Part model, mm, in its own coordinate system. Round coordinates to 2 decimals unless told otherwise and drop trailing zeros. Write each loop counter-clockwise with the first axis right and the second up, starting at its lowest first coordinate (ties: lowest second). Pieces come first, ordered by that corner, then holes. Notation, with made-up numbers: M 19,-36.75 L 48,-36.75 A22 ccw 48,-26.75 Z; hole C -17,84 d10. An arc over 180 degrees is marked long. Answer as a JSON object with one key per item and string values. Group by question number.
1. Two-plate mould, pull along X, no slides. Class faces 1 (the face through (-44.05, -198.368, 9.392)), 2 (the face through (-114, 171, 0)), 3 (the face through (-55.06, -247.96, 9.39)): +X half, -X half, draft (parallel to the pull), parting line (faces both ways), or undercut.
2. Band-saw the part on C-C, the plane z = 12.5. Write the cut outline in (x, y) (3 decimals), plus the area to 3 significant figures.
3. Drill centre lines: line 1 (Y direction, x = 0, z = 12.75); line 2 (X direction, y = -141.5, z = 11.25); line 3 (X direction, y = 89.5, z = 15.5). Where is each one in solid material? Low to high. Write a range as from..to.
4. Band-saw the part on D-D, the plane y = -220. Write the cut outline in (x, z).
5. Drop flat-ended pins along their axis: pin 1 (8 mm diameter, centred on y = -112, z = 15, fed in from +X); pin 2 (2 mm diameter, centred on y = 44, z = 4, fed in from -X); pin 3 (10 mm diameter, centred on x = -197.5, y = 8.5, fed in from +Z); pin 4 (1 mm diameter, centred on x = 125, z = 8.5, fed in from +Y) (3 decimals). Give the stop position or say it passes through.
6. Band-saw the part on A-A, the plane y = 0. Write the cut outline in (x, z), plus the area to 3 significant figures.
from build123d import *

# Parameters (mm, degrees)
F0_R     = 254
F0_R_2   = 203.2
F1_DEPTH = 19.05


with BuildPart() as f1:
    # F0 (on Top) → F1 (new body)
    with BuildSketch(Plane.XY):
        Circle(F0_R)
        with BuildLine():
            ThreePointArc((196.7011125508, 128.4919251209), (225.1848450649, 67.0319927579), (234.95, 0))
            ThreePointArc((234.95, 0), (229.2479499847, -51.4478369596), (212.4185683948, -100.3984775836))
            ThreePointArc((212.4185683948, -100.3984775836), (213.7303800146, -101.5698688542), (214.2174677682, -103.259766116))
            ThreePointArc((214.2174677682, -103.259766116), (212.7141648851, -105.9590352298), (209.6278276113, -106.1021978612))
            ThreePointArc((209.6278276113, -106.1021978612), (131.1382553066, -194.9468145294), (19.2616521087, -234.1591152572))
            ThreePointArc((19.2616521087, -234.1591152572), (19.2684021583, -234.2784835874), (19.2706532388, -234.3980214226))
            ThreePointArc((19.2706532388, -234.3980214226), (16.1937508526, -237.5715056053), (12.9267150604, -234.5941229821))
            ThreePointArc((12.9267150604, -234.5941229821), (-103.259766116, -211.0424677682), (-193.1569162861, -133.7606376736))
            ThreePointArc((-193.1569162861, -133.7606376736), (-197.5812309419, -132.9103938918), (-196.7011125508, -128.4919251209))
            ThreePointArc((-196.7011125508, -128.4919251209), (-234.3980214226, -16.0956532388), (-212.4185683948, 100.3984775836))
            ThreePointArc((-212.4185683948, 100.3984775836), (-213.8943930083, 104.6551683608), (-209.6278276113, 106.1021978612))
            ThreePointArc((-209.6278276113, 106.1021978612), (-131.1382553066, 194.9468145294), (-19.2616521087, 234.1591152572))
            ThreePointArc((-19.2616521087, 234.1591152572), (-16.3131620664, 237.5655622526), (-12.9267150604, 234.5941229821))
            ThreePointArc((-12.9267150604, 234.5941229821), (103.259766116, 211.0424677682), (193.1569162861, 133.7606376736))
            ThreePointArc((193.1569162861, 133.7606376736), (196.4296661871, 133.9457053883), (198.1218145294, 131.1382553066))
            ThreePointArc((198.1218145294, 131.1382553066), (197.744181257, 129.6364682408), (196.7011125508, 128.4919251209))
        make_face(mode=Mode.SUBTRACT)
        with BuildLine():
            ThreePointArc((212.4185683948, -100.3984775836), (229.2479499847, -51.4478369596), (234.95, 0))
            ThreePointArc((234.95, 0), (225.1848450649, 67.0319927579), (196.7011125508, 128.4919251209))
            ThreePointArc((196.7011125508, 128.4919251209), (192.3123981168, 129.3661167214), (193.1569162861, 133.7606376736))
            ThreePointArc((193.1569162861, 133.7606376736), (103.259766116, 211.0424677682), (-12.9267150604, 234.5941229821))
            ThreePointArc((-12.9267150604, 234.5941229821), (-12.9221690561, 234.4961190364), (-12.9206532388, 234.3980214226))
            ThreePointArc((-12.9206532388, 234.3980214226), (-15.9761154036, 231.2252725031), (-19.2616521087, 234.1591152572))
            ThreePointArc((-19.2616521087, 234.1591152572), (-131.1382553066, 194.9468145294), (-209.6278276113, 106.1021978612))
            ThreePointArc((-209.6278276113, 106.1021978612), (-208.3431986543, 104.931463233), (-207.8674677682, 103.259766116))
            ThreePointArc((-207.8674677682, 103.259766116), (-209.3525705064, 100.5718538695), (-212.4185683948, 100.3984775836))
            ThreePointArc((-212.4185683948, 100.3984775836), (-234.3980214226, -16.0956532388), (-196.7011125508, -128.4919251209))
            ThreePointArc((-196.7011125508, -128.4919251209), (-193.4450274636, -128.3408885789), (-191.7718145294, -131.1382553066))
            ThreePointArc((-191.7718145294, -131.1382553066), (-192.1393644477, -132.6211069643), (-193.1569162861, -133.7606376736))
            ThreePointArc((-193.1569162861, -133.7606376736), (-103.259766116, -211.0424677682), (12.9267150604, -234.5941229821))
            ThreePointArc((12.9267150604, -234.5941229821), (15.8781444113, -231.2304805925), (19.2616521087, -234.1591152572))
            ThreePointArc((19.2616521087, -234.1591152572), (131.1382553066, -194.9468145294), (209.6278276113, -106.1021978612))
            ThreePointArc((209.6278276113, -106.1021978612), (208.190542528, -101.8643638712), (212.4185683948, -100.3984775836))
        make_face()
        Circle(F0_R_2, mode=Mode.SUBTRACT)
    extrude(amount=F1_DEPTH)


solid = f1.part
Worked answers:
{
 "1": {"face 1": "undercut", "face 2": "draft", "face 3": "parting line"},
 "2": {"outline": "C 0,0 d508; hole C -211.042,103.26 d6.35; hole C 0,0 d406.4; hole C -194.947,-131.138 d6.35; hole C -16.096,234.398 d6.35; hole C 16.096,-234.398 d6.35; hole C 194.947,131.138 d6.35; hole C 211.042,-103.26 d6.35", "area": "72,800 mm^2"},
 "3": {"line 1": "y = -254..-203.2, 203.2..254", "line 2": "x = -210.94..-145.84, 145.84..210.94", "line 3": "x = -237.71..-182.43, 182.43..237.71"},
 "4": {"outline": "M -126.95,0 L 126.95,0 L 126.95,19.05 L -126.95,19.05 Z"},
 "5": {"pin 1": "stops at x = 229.9", "pin 2": "stops at x = -250.33", "pin 3": "passes through", "pin 4": "stops at y = 221.395"},
 "6": {"outline": "M -254,0 L -203.2,0 L -203.2,19.05 L -254,19.05 Z; M 203.2,0 L 254,0 L 254,19.05 L 203.2,19.05 Z", "area": "1,940 mm^2"}
}
